Check sheet for the modelled part. Datum: model origin and axes. Units: mm. Give positions to 0.01 mm unless a question says otherwise; leave off trailing zeros. Order: outer loops, then holes, each group sorted by start corner. A loop starts at its lowest first (then second) coordinate and runs counter-clockwise, first axis right, second up.
from build123d import *

# Parameters (mm, degrees)
BOSS_EXTRUDE1_DEPTH = 6
SKETCH9_R           = 5.691956205
SKETCH9_R_2         = 5.691972425
SKETCH9_R_3         = 5.691961612
CUT_EXTRUDE1_DEPTH  = 6
SCALE2_SCALE        = 0.3527


with BuildPart() as part:
    # Sketch8 → Boss-Extrude1 (new body)
    with BuildSketch(Plane.XY):
        Polygon((455.046069669, 138.815328461), (455.046069669, 461.140101754), (418.818767583, 461.140101754), (417.854464359, 491.424711157), (389.623159284, 491.424711157), (389.623159284, 519.966114473), (276.778792345, 519.966114473), (276.778792345, 489.453304052), (246.138948372, 489.453304052), (246.138948372, 462.665142262), (209.772989289, 462.665142262), (209.772989289, 138.815328461), align=None)
        Polygon((352.800007218, 274.896015056), (320.400005452, 274.896015056), (320.400005452, 255.096012775), (315.000008762, 255.096012775), (315.000008762, 188.496024764), (358.200003908, 188.496024764), (358.200003908, 253.29600667), (352.800007218, 253.29600667), align=None, mode=Mode.SUBTRACT)
    extrude(amount=BOSS_EXTRUDE1_DEPTH)

    # Sketch9 → Cut-Extrude1 (cut)
    with BuildSketch(Plane(origin=(0, 0, 0), x_dir=(-1, 0, 0), z_dir=(0, 0, -1))):
        with Locations((-442.800031348, 150.987964196)):
            Circle(SKETCH9_R)
        with Locations((-256.719699101, 478.692872416)):
            Circle(SKETCH9_R_2)
        with Locations((-406.119708447, 480.492867708)):
            Circle(SKETCH9_R_3)
    extrude(amount=-CUT_EXTRUDE1_DEPTH, mode=Mode.SUBTRACT)


with BuildPart() as part_1:
    # Scale2: scaled about (332.105882885, 321.548539841, 3)
    add(part.part.scale(SCALE2_SCALE).moved(Location((214.972137991, 208.138369839, 1.9419))))


solid = part_1.part
1) Section check A-A, the plane x = 332. Record the cut outline in (y, z).
Recorded:
outline: (257.1, 1.94) - (274.62, 1.94) - (274.62, 4.06) - (257.1, 4.06) - close; (305.09, 1.94) - (391.53, 1.94) - (391.53, 4.06) - (305.09, 4.06) - close
2) Section check D-D, the plane x = 367. Record the cut outline in (y, z).
Recorded:
outline: (257.1, 1.94) - (370.78, 1.94) - (370.78, 4.06) - (257.1, 4.06) - close
3) Draft check along X on faces 1 (the face through (356.296, 378.211, 2.985)), 2 (the face through (332, 325, 1.942)), 3 (the face through (307.11, 375.75, 2.99)). Enter one of: +X half, -X half, draft (parallel to the pull), parting line (faces both ways), or undercut.
Recorded:
face 1: undercut
face 2: draft
face 3: undercut
4) Section check C-C, the plane z = 2.5. Record the cut outline in (x, y), then the cut area to 3 significant figures.
Recorded:
outline: (288.96, 257.1) - (375.47, 257.1) - (375.47, 370.78) - (362.69, 370.78) - (362.35, 381.46) - (352.39, 381.46) - (352.39, 391.53) - (312.59, 391.53) - (312.59, 380.77) - (301.79, 380.77) - (301.79, 371.32) - (288.96, 371.32) - close; hole circle Ø4.02 at (305.52, 376.97); hole (326.07, 274.62) - (341.31, 274.62) - (341.31, 297.48) - (339.4, 297.48) - (339.4, 305.09) - (327.98, 305.09) - (327.98, 298.11) - (326.07, 298.11) - close; hole circle Ø4.02 at (358.21, 377.61); hole circle Ø4.02 at (371.15, 261.39)
area: 10,400 mm2
5) Section check B-B, the plane y = 285. Record the cut outline in (x, z), then the cut area to 3 significant figures.
Recorded:
outline: (288.96, 1.94) - (326.07, 1.94) - (326.07, 4.06) - (288.96, 4.06) - close; (341.31, 1.94) - (375.47, 1.94) - (375.47, 4.06) - (341.31, 4.06) - close
area: 151 mm2
6) Material ranges on L1, parallel to X at y = 376, z = 3.75; L2, parallel to X at y = 293.5, z = 2.45; L3, parallel to Y at x = 353, z = 2.4, recorded low to high.
Recorded:
L1: x = 301.79 to 303.76, 307.27 to 357.01, 359.41 to 362.52
L2: x = 288.96 to 326.07, 341.31 to 375.47
L3: y = 257.1 to 381.46
7) Depth check by flat-ended pin: pin 1 Ø0.6 at (x, z) = (294.5, 3.5) entering from +Y; pin 2 Ø1.1 at (y, z) = (375.5, 3) entering from -X; pin 3 Ø1.1 at (y, z) = (384.5, 3) entering from -X. Enter the tip coordinate at first touch or a pass-through.
Recorded:
pin 1: stops at y = 371.32
pin 2: stops at x = 301.79
pin 3: stops at x = 312.59
